from build123d import *

# Parameters (mm, degrees)
MAIN_BODY_DEPTH     = 6.35
RASPBERRY_PI_REACH  = 122.169
SKETCH2_R           = 1.025
MOTOR_MOUNTS_REACH  = 122.169
SKETCH3_R           = 1.143
CUT_EXTRUDE3_REACH  = 122.169
SKETCH4_R           = 1.143
SKETCH5_R           = 1.143
GRABBER_MOUNT_DEPTH = 121.168600308
SKETCH6_R           = 1.143
FRONT_IR_DEPTH      = 121.168600308
SKETCH8_R           = 1.143
SIDE_IR_DEPTH       = 121.168600308
SKETCH9_R           = 1.143
CUT_EXTRUDE4_DEPTH  = 121.168600308
SKETCH10_W          = 38.1
SKETCH10_H          = 25.908
CUT_EXTRUDE5_DEPTH  = 121.168600308


with BuildPart() as part:
    # Sketch1 → Main Body (new body)
    with BuildSketch(Plane(origin=(0, 0, 0), x_dir=(1, 0, 0), z_dir=(0, 1, 0))):
        with BuildLine():
            Line((-80.603721998, 37.5), (-80.603721998, -37.5))
            ThreePointArc((-80.603721998, -37.5), (0, -88.9), (80.603721998, -37.5))
            Line((80.603721998, -37.5), (80.603721998, 37.5))
            ThreePointArc((80.603721998, 37.5), (0, 88.9), (-80.603721998, 37.5))
        make_face()
    extrude(amount=MAIN_BODY_DEPTH)

    # Sketch2 → Raspberry Pi (cut, up to next)
    with BuildSketch(Plane(origin=(0, 6.35, 0), x_dir=(1, 0, 0), z_dir=(0, 1, 0)), mode=Mode.PRIVATE) as raspberry_pi_sk1:
        with Locations(Location((24.5, 69.85, 0), (0, 0, 270))):
            Circle(SKETCH2_R)
    raspberry_pi_tool1 = extrude(raspberry_pi_sk1.sketch, amount=-RASPBERRY_PI_REACH, mode=Mode.PRIVATE) & part.part
    # Sketch2 → Raspberry Pi (cut, up to next)
    with BuildSketch(Plane(origin=(0, 6.35, 0), x_dir=(1, 0, 0), z_dir=(0, 1, 0)), mode=Mode.PRIVATE) as raspberry_pi_sk2:
        with Locations(Location((24.5, 11.85, 0), (0, 0, 270))):
            Circle(SKETCH2_R)
    raspberry_pi_tool2 = extrude(raspberry_pi_sk2.sketch, amount=-RASPBERRY_PI_REACH, mode=Mode.PRIVATE) & part.part
    # Sketch2 → Raspberry Pi (cut, up to next)
    with BuildSketch(Plane(origin=(0, 6.35, 0), x_dir=(1, 0, 0), z_dir=(0, 1, 0)), mode=Mode.PRIVATE) as raspberry_pi_sk3:
        with Locations(Location((-24.5, 11.85, 0), (0, 0, 270))):
            Circle(SKETCH2_R)
    raspberry_pi_tool3 = extrude(raspberry_pi_sk3.sketch, amount=-RASPBERRY_PI_REACH, mode=Mode.PRIVATE) & part.part
    # Sketch2 → Raspberry Pi (cut, up to next)
    with BuildSketch(Plane(origin=(0, 6.35, 0), x_dir=(1, 0, 0), z_dir=(0, 1, 0)), mode=Mode.PRIVATE) as raspberry_pi_sk4:
        with Locations(Location((-24.5, 69.85, 0), (0, 0, 270))):
            Circle(SKETCH2_R)
    raspberry_pi_tool4 = extrude(raspberry_pi_sk4.sketch, amount=-RASPBERRY_PI_REACH, mode=Mode.PRIVATE) & part.part
    add(raspberry_pi_tool1.solids().sort_by_distance((24.5, 6.35, -69.85))[0], mode=Mode.SUBTRACT)
    add(raspberry_pi_tool2.solids().sort_by_distance((24.5, 6.35, -11.85))[0], mode=Mode.SUBTRACT)
    add(raspberry_pi_tool3.solids().sort_by_distance((-24.5, 6.35, -11.85))[0], mode=Mode.SUBTRACT)
    add(raspberry_pi_tool4.solids().sort_by_distance((-24.5, 6.35, -69.85))[0], mode=Mode.SUBTRACT)

    # Sketch3 → Motor Mounts (cut, up to next)
    with BuildSketch(Plane(origin=(0, 6.35, 0), x_dir=(1, 0, 0), z_dir=(0, 1, 0)), mode=Mode.PRIVATE) as motor_mounts_sk1:
        with Locations(Location((-74.353721998, 9, 0), (0, 0, 270))):
            Circle(SKETCH3_R)
    motor_mounts_tool1 = extrude(motor_mounts_sk1.sketch, amount=-MOTOR_MOUNTS_REACH, mode=Mode.PRIVATE) & part.part
    # Sketch3 → Motor Mounts (cut, up to next)
    with BuildSketch(Plane(origin=(0, 6.35, 0), x_dir=(1, 0, 0), z_dir=(0, 1, 0)), mode=Mode.PRIVATE) as motor_mounts_sk2:
        with Locations(Location((-74.353721998, -9, 0), (0, 0, 270))):
            Circle(SKETCH3_R)
    motor_mounts_tool2 = extrude(motor_mounts_sk2.sketch, amount=-MOTOR_MOUNTS_REACH, mode=Mode.PRIVATE) & part.part
    # Sketch3 → Motor Mounts (cut, up to next)
    with BuildSketch(Plane(origin=(0, 6.35, 0), x_dir=(1, 0, 0), z_dir=(0, 1, 0)), mode=Mode.PRIVATE) as motor_mounts_sk3:
        with Locations(Location((74.353721998, 9, 0), (0, 0, 270))):
            Circle(SKETCH3_R)
    motor_mounts_tool3 = extrude(motor_mounts_sk3.sketch, amount=-MOTOR_MOUNTS_REACH, mode=Mode.PRIVATE) & part.part
    # Sketch3 → Motor Mounts (cut, up to next)
    with BuildSketch(Plane(origin=(0, 6.35, 0), x_dir=(1, 0, 0), z_dir=(0, 1, 0)), mode=Mode.PRIVATE) as motor_mounts_sk4:
        with Locations(Location((74.353721998, -9, 0), (0, 0, 270))):
            Circle(SKETCH3_R)
    motor_mounts_tool4 = extrude(motor_mounts_sk4.sketch, amount=-MOTOR_MOUNTS_REACH, mode=Mode.PRIVATE) & part.part
    add(motor_mounts_tool1.solids().sort_by_distance((-74.353722, 6.35, -9))[0], mode=Mode.SUBTRACT)
    add(motor_mounts_tool2.solids().sort_by_distance((-74.353722, 6.35, 9))[0], mode=Mode.SUBTRACT)
    add(motor_mounts_tool3.solids().sort_by_distance((74.353722, 6.35, -9))[0], mode=Mode.SUBTRACT)
    add(motor_mounts_tool4.solids().sort_by_distance((74.353722, 6.35, 9))[0], mode=Mode.SUBTRACT)

    # Sketch4 → Cut-Extrude3 (cut, up to next)
    with BuildSketch(Plane(origin=(0, 6.35, 0), x_dir=(1, 0, 0), z_dir=(0, 1, 0)), mode=Mode.PRIVATE) as cut_extrude3_sk1:
        with Locations(Location((-7.747, 78.9, 0), (0, 0, 270))):
            Circle(SKETCH4_R)
    cut_extrude3_tool1 = extrude(cut_extrude3_sk1.sketch, amount=-CUT_EXTRUDE3_REACH, mode=Mode.PRIVATE) & part.part
    # Sketch4 → Cut-Extrude3 (cut, up to next)
    with BuildSketch(Plane(origin=(0, 6.35, 0), x_dir=(1, 0, 0), z_dir=(0, 1, 0)), mode=Mode.PRIVATE) as cut_extrude3_sk2:
        with Locations(Location((7.747, 78.9, 0), (0, 0, 270))):
            Circle(SKETCH4_R)
    cut_extrude3_tool2 = extrude(cut_extrude3_sk2.sketch, amount=-CUT_EXTRUDE3_REACH, mode=Mode.PRIVATE) & part.part
    add(cut_extrude3_tool1.solids().sort_by_distance((-7.747, 6.35, -78.9))[0], mode=Mode.SUBTRACT)
    add(cut_extrude3_tool2.solids().sort_by_distance((7.747, 6.35, -78.9))[0], mode=Mode.SUBTRACT)

    # Sketch5 → Grabber Mount (cut, through all)
    with BuildSketch(Plane(origin=(0, 6.35, 0), x_dir=(1, 0, 0), z_dir=(0, 1, 0))):
        with Locations(Location((35.56, -24.48608666, 0), (0, 0, 270))):
            Circle(SKETCH5_R)
        with Locations(Location((35.56, -72.74608666, 0), (0, 0, 270))):
            Circle(SKETCH5_R)
    extrude(amount=-GRABBER_MOUNT_DEPTH, mode=Mode.SUBTRACT)

    # Sketch6 → Front IR (cut, through all)
    with BuildSketch(Plane(origin=(0, 6.35, 0), x_dir=(1, 0, 0), z_dir=(0, 1, 0))):
        with Locations(Location((-12.7, -69.596, 0), (0, 0, 270))):
            Circle(SKETCH6_R)
        with Locations(Location((12.7, -69.596, 0), (0, 0, 270))):
            Circle(SKETCH6_R)
    extrude(amount=-FRONT_IR_DEPTH, mode=Mode.SUBTRACT)

    # Sketch8 → Side IR (cut, through all)
    with BuildSketch(Plane(origin=(0, 6.35, 0), x_dir=(1, 0, 0), z_dir=(0, 1, 0))):
        with Locations(Location((-63.5, -37.5, 0), (0, 0, 270))):
            Circle(SKETCH8_R)
        with Locations(Location((-63.5, -50.2, 0), (0, 0, 270))):
            Circle(SKETCH8_R)
        with Locations(Location((63.5, -50.2, 0), (0, 0, 90))):
            Circle(SKETCH8_R)
        with Locations(Location((63.5, -37.5, 0), (0, 0, 90))):
            Circle(SKETCH8_R)
    extrude(amount=-SIDE_IR_DEPTH, mode=Mode.SUBTRACT)

    # Sketch9 → Cut-Extrude4 (cut, through all)
    with BuildSketch(Plane(origin=(0, 6.35, 0), x_dir=(1, 0, 0), z_dir=(0, 1, 0))):
        with Locations(Location((-55.203721998, -25.62908666, 0), (0, 0, 270))):
            Circle(SKETCH9_R)
        with Locations(Location((-17.103721998, -25.62908666, 0), (0, 0, 270))):
            Circle(SKETCH9_R)
    extrude(amount=-CUT_EXTRUDE4_DEPTH, mode=Mode.SUBTRACT)

    # Sketch10 → Cut-Extrude5 (cut, through all)
    with BuildSketch(Plane(origin=(0, 6.35, 0), x_dir=(1, 0, 0), z_dir=(0, 1, 0))):
        with Locations((0, -88.9)):
            Rectangle(SKETCH10_W, SKETCH10_H)
    extrude(amount=-CUT_EXTRUDE5_DEPTH, mode=Mode.SUBTRACT)


solid = part.part
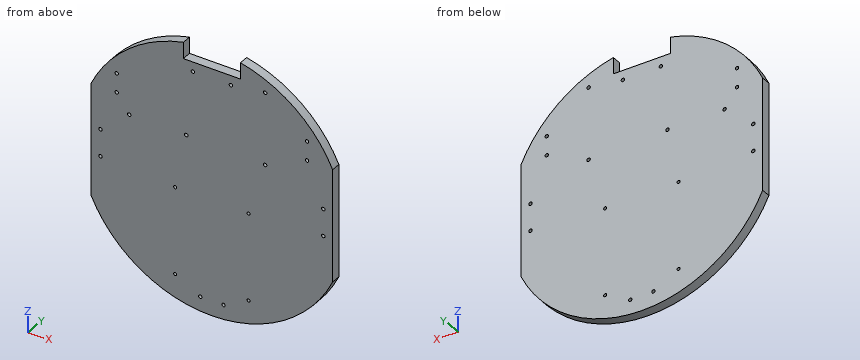
Geometry check sheet. Reference: the model listing, model coordinates, mm. Give positions to 0.01 mm unless a question says otherwise; leave off trailing zeros. Loops run counter-clockwise (first coordinate to the right, second up) from the corner with the lowest first, then second, coordinate; pieces in that order, holes last. Notation, with made-up numbers: M 51.5,-7 L 61.5,-7 A24 ccw 61.5,8 Z; hole C 15.5,66.25 d4. An arc over 180 degrees is marked long. Answer as a JSON object with one key per item and string values. Group by question number.
Item 1: Sectioned sample at B-B on z = -44. Record the boundary of the cut face in (x, y).
Item 2: Sectioned sample at A-A on y = 4. Give the number of separate pieces and of enclosed holes in the cut face, plus the area to 3 significant figures.
Item 3: Material ranges on L1, parallel to X at y = 3, z = -11.85 (3 decimals); L2, parallel to X at y = 1.75, z = -78; L3, parallel to Z at x = -24, y = 4, recorded low to high.
Item 4: Gauge pin test, flat ends, axial feed: pin 1 (3.5 mm diameter, centred on x = 63.5, z = 37.5, fed in from -Y); pin 2 (2 mm diameter, centred on x = -30, y = 3, fed in from -Z); pin 3 (3 mm diameter, centred on x = -59, y = 4, fed in from +Z); pin 4 (1.9 mm diameter, centred on y = 1.5, z = 79, fed in from +X). Record the tip position at first contact, or that the pin passes through.
Findings below:
{
 "1": {"outline": "M -77.25,0 L 77.25,0 L 77.25,6.35 L -77.25,6.35 Z"},
 "2": {"separate pieces": "1", "enclosed holes": "20", "area": "23,400 mm2"},
 "3": {"L1": "-80.604 to -25.525, -23.475 to 23.475, 25.525 to 80.604", "L2": "-42.65 to -8.45, -7.04 to 7.04, 8.45 to 42.65", "L3": "-85.6 to -70.74, -68.96 to -12.74, -10.96 to 85.6"},
 "4": {"pin 1": "y = 0", "pin 2": "z = -84.04", "pin 3": "z = 67.8", "pin 4": "x = 42.56"}
}
